from build123d import *

# Parameters (mm, degrees)
SKETCH1_R           = 35
SKETCH2_R           = 5.224283628
SKETCH8_R           = 5.224283628
BOSS_EXTRUDE1_DEPTH = 10
SKETCH16_W          = 13
SKETCH16_H          = 33
BOSS_EXTRUDE5_DEPTH = 1.5
SKETCH19_R          = 4.5
BOSS_EXTRUDE6_DEPTH = 13
SKETCH21_W          = 9
SKETCH21_H          = 108.66
BOSS_EXTRUDE7_DEPTH = 6.5
SKETCH22_R          = 35
BOSS_EXTRUDE8_DEPTH = 2
SKETCH23_R          = 15
BOSS_EXTRUDE9_DEPTH = 5


with BuildPart() as part:
    # Sketch1 → Loft3 section 0
    with BuildSketch(Plane(origin=(0, 0, 0), x_dir=(1, 0, 0), z_dir=(0, 1, 0))):
        Circle(SKETCH1_R)
    # Sketch2 → Loft3 section 1
    with BuildSketch(Plane(origin=(0, 10, 0), x_dir=(1, 0, 0), z_dir=(0, 1, 0))):
        Circle(SKETCH2_R)
    loft()

    # Sketch8 → Boss-Extrude1 (add)
    with BuildSketch(Plane(origin=(0, 10, 0), x_dir=(1, 0, 0), z_dir=(0, 1, 0))):
        with Locations(Location((0, 0, 0), (0, 0, 90))):
            Circle(SKETCH8_R)
    extrude(amount=BOSS_EXTRUDE1_DEPTH)

    # Sketch16 → Boss-Extrude5 (add, symmetric)
    with BuildSketch(Plane.XY.offset(10)):
        with Locations((-18.340938927, 16.5)):
            Rectangle(SKETCH16_W, SKETCH16_H)
    boss_extrude5 = extrude(amount=BOSS_EXTRUDE5_DEPTH, both=True)

    # Mirror2: Boss-Extrude5 across plane
    add(boss_extrude5.mirror(Plane.XY))

    # Sketch19 → Boss-Extrude6 (add, symmetric)
    with BuildSketch(Plane.XY):
        with Locations(Location((-18.340938927, 24.342530905, 0), (0, 0, 180))):
            Circle(SKETCH19_R)
    extrude(amount=BOSS_EXTRUDE6_DEPTH, both=True)

    # Sketch21 → Boss-Extrude7 (add, symmetric)
    with BuildSketch(Plane.XY):
        with Locations((-18.340938927, 78.672530905)):
            Rectangle(SKETCH21_W, SKETCH21_H)
    extrude(amount=BOSS_EXTRUDE7_DEPTH, both=True)

    # Sketch22 → Boss-Extrude8 (add)
    with BuildSketch(Plane(origin=(0, 0, 0), x_dir=(1, 0, 0), z_dir=(0, 1, 0))):
        with Locations(Location((0, 0, 0), (0, 0, 270))):
            Circle(SKETCH22_R)
    extrude(amount=-BOSS_EXTRUDE8_DEPTH)

    # Sketch23 → Boss-Extrude9 (add)
    with BuildSketch(Plane(origin=(0, 133.002530905, 0), x_dir=(1, 0, 0), z_dir=(0, 1, 0))):
        with Locations(Location((-18.340938927, 0, 0), (0, 0, 270))):
            Circle(SKETCH23_R)
    extrude(amount=BOSS_EXTRUDE9_DEPTH)


solid = part.part
Check sheet for the modelled part. Datum: model origin and axes. Units: mm. A direction names the side the tool comes from. Coordinates: 2 decimals unless noted, no trailing zeros. Write each loop counter-clockwise with the first axis right and the second up, starting at its lowest first coordinate (ties: lowest second). Pieces come first, ordered by that corner, then holes.
Item 1: Scan lines: probe 1 along Z at (x, y) = (-16, 15); probe 2 along Y at (x, z) = (-19.5, -9.5); probe 3 along Z at (x, y) = (-16, 125). Record each from-to range of solid material in increasing order.
Numbers:
probe 1: z = -11.5 to -8.5, 8.5 to 11.5
probe 2: y = -2 to 33, 133 to 138
probe 3: z = -6.5 to 6.5
Item 2: Mould release check, pull along Y, two halves, no side actions. Record for faces 1 (the face through (-18, 138.003, 0)), 2 (the face through (-13.841, 78, 0)), 3 (the face through (-32.984, 135.468, -3.252)): released by +Y, released by -Y, zero draft, split by the parting line, or undercut.
Numbers:
face 1: released by +Y
face 2: undercut
face 3: zero draft
Item 3: Cross-section at C-C on y = 26. Record the boundary of the cut face in (x, z), then the cut area to 3 significant figures.
Numbers:
outline: (-24.84, -11.5) - (-22.52, -11.5) - (-22.52, -13) - (-14.16, -13) - (-14.16, -11.5) - (-11.84, -11.5) - (-11.84, -8.5) - (-14.16, -8.5) - (-14.16, -6.5) - (-13.84, -6.5) - (-13.84, 6.5) - (-14.16, 6.5) - (-14.16, 8.5) - (-11.84, 8.5) - (-11.84, 11.5) - (-14.16, 11.5) - (-14.16, 13) - (-22.52, 13) - (-22.52, 11.5) - (-24.84, 11.5) - (-24.84, 8.5) - (-22.52, 8.5) - (-22.52, 6.5) - (-22.84, 6.5) - (-22.84, -6.5) - (-22.52, -6.5) - (-22.52, -8.5) - (-24.84, -8.5) - close
area: 254 mm2
Item 4: Cross-section at B-B on y = 121. Record the boundary of the cut face in (x, z).
Numbers:
outline: (-22.84, -6.5) - (-13.84, -6.5) - (-13.84, 6.5) - (-22.84, 6.5) - close
Item 5: Access from +Z, -Z, +X, -X, +Y, -Y to the whole of each face (thin tool, end or side, straight path). Record for faces 4 (the face through (-18, 24, 13)), 5 (the face through (0, 20, 0)), 6 (the face through (-14.77, 27.08, -12.24)), 7 (the face through (-18, 24, -13)), 8 (the face through (5.1, 14.93, 1.13)).
Numbers:
face 4: +Z, +X, -X
face 5: +Z, -Z, +X
face 6: -Z
face 7: -Z, +X, -X
face 8: none
Item 6: Cross-section at A-A on x = 0. Record the boundary of the cut face in (y, z), then the cut area to 3 significant figures.
Numbers:
outline: (-2, -35) - (0, -35) - (10, -5.22) - (20, -5.22) - (20, 5.22) - (10, 5.22) - (0, 35) - (-2, 35) - close
area: 647 mm2
Item 7: Depth check by flat-ended pin: pin 1 Ø2.5 at (x, y) = (-20, 92) entering from +Z; pin 2 Ø14.5 at (x, y) = (-19, 17.5) entering from +Z; pin 3 Ø4.5 at (x, y) = (-20, 24) entering from -Z. Enter the tip coordinate at first touch or a pass-through.
Numbers:
pin 1: stops at z = 6.5
pin 2: stops at z = 13
pin 3: stops at z = -13
